Design review of the part built by this model. Coordinates are the model's own, in mm. Coordinates: 2 decimals unless noted, no trailing zeros. Loops run counter-clockwise (first coordinate to the right, second up) from the corner with the lowest first, then second, coordinate; pieces in that order, holes last. Notation, with made-up numbers: (79.5, 39.5) -> (96.5, 39.5) arc R12 ccw to (96.5, 52.5) -> close; hole circle Ø3 at (-18, 17.5). An arc over 180 degrees is marked (long way). One line per item, written item: value. Start each with the question number.
1. Insertion check: pin 1 (2 mm diameter, centred on y = 1.5, z = -86.5, fed in from -X); pin 2 (3 mm diameter, centred on x = 107, y = -1, fed in from -Z); pin 3 (3 mm diameter, centred on y = 1, z = 0, fed in from +X); pin 4 (1.8 mm diameter, centred on x = 64.87, z = 64.87, fed in from -Y). Each pin has a flat end and moves straight along its axis. Give the tip position at first contact, or say it passes through.
2. Add section C-C on y = 1.25. Give the number of separate pieces and of enclosed holes in the cut face, plus the area to 3 significant figures.
3. For probe 1 along Z at (x, y) = (-51.5, 0.75); probe 2 along Z at (x, y) = (33, -3); probe 3 along X at (y, z) = (0, 36.5), list the stretches that pass through material, from the lowest coordinate up.
4. Add section A-A on z = 55. Write out the cut boundary in (x, y) (3 decimals).
5. Add section B-B on x = -29. Write out the cut boundary in (y, z) (3 decimals), plus the area to 3 significant figures.
```python
from build123d import *

# Parameters (mm, degrees)
BOSS_EXTRUDE1_DEPTH          = 3.175
SKETCH2_W                    = 2.75
SKETCH2_H                    = 2.5
SKETCH2_H_2                  = 4
SKETCH2_W_2                  = 1.125
SKETCH2_H_3                  = 7.5
CUT_EXTRUDE1_DEPTH           = 230.978807609
CIRPATTERN1_COUNT            = 4
F_3_0_3_DIAMETER_HOLE1_D     = 3
F_8_0_8_DIAMETER_HOLE1_D     = 8
F_8_0_8_DIAMETER_HOLE1_DEPTH = 6.35


with BuildPart() as part:
    # Sketch1 → Boss-Extrude1 (new, symmetric)
    with BuildSketch(Plane(origin=(0, 0, 0), x_dir=(1, 0, 0), z_dir=(0, 1, 0))):
        with BuildLine():
            Line((88.388347648, 98.994949366), (64.667874078, 75.274475795))
            ThreePointArc((64.667874078, 75.274475795), (-70.171862751, 70.171862751), (-75.274475795, -64.667874078))
            Line((-75.274475795, -64.667874078), (-98.994949366, -88.388347648))
            Line((-98.994949366, -88.388347648), (-54.800775542, -132.582521472))
            ThreePointArc((-54.800775542, -132.582521472), (17.67766953, -162.604076401), (90.156114601, -132.582521472))
            Line((90.156114601, -132.582521472), (132.582521472, -90.156114601))
            ThreePointArc((132.582521472, -90.156114601), (162.604076401, -17.67766953), (132.582521472, 54.800775542))
            Line((132.582521472, 54.800775542), (88.388347648, 98.994949366))
        make_face()
        with BuildLine():
            Line((-7.5, -7.5), (-7.5, -83.903460262))
            ThreePointArc((-7.5, -83.903460262), (-59.565261034, -59.565261034), (-83.903460262, -7.5))
            Line((-83.903460262, -7.5), (-7.5, -7.5))
        make_face(mode=Mode.SUBTRACT)
        with BuildLine():
            ThreePointArc((83.903460262, -7.5), (59.565261034, -59.565261034), (7.5, -83.903460262))
            Line((7.5, -83.903460262), (7.5, -7.5))
            Line((7.5, -7.5), (83.903460262, -7.5))
        make_face(mode=Mode.SUBTRACT)
        with BuildLine():
            ThreePointArc((-64.667874078, -75.274475795), (0, -99.238), (64.667874078, -75.274475795))
            Line((64.667874078, -75.274475795), (95.45941546, -106.066017178))
            Line((95.45941546, -106.066017178), (79.549512883, -121.975919755))
            ThreePointArc((79.549512883, -121.975919755), (17.67766953, -147.604076401), (-44.194173824, -121.975919755))
            Line((-44.194173824, -121.975919755), (-77.781745931, -88.388347648))
            Line((-77.781745931, -88.388347648), (-64.667874078, -75.274475795))
        make_face(mode=Mode.SUBTRACT)
        with BuildLine():
            ThreePointArc((75.274475795, -64.667874078), (99.238, 0), (75.274475795, 64.667874078))
            Line((75.274475795, 64.667874078), (88.388347648, 77.781745931))
            Line((88.388347648, 77.781745931), (121.975919755, 44.194173824))
            ThreePointArc((121.975919755, 44.194173824), (147.604076401, -17.67766953), (121.975919755, -79.549512883))
            Line((121.975919755, -79.549512883), (106.066017178, -95.45941546))
            Line((106.066017178, -95.45941546), (75.274475795, -64.667874078))
        make_face(mode=Mode.SUBTRACT)
        with BuildLine():
            Line((-7.5, 7.5), (-83.903460262, 7.5))
            ThreePointArc((-83.903460262, 7.5), (-59.565261034, 59.565261034), (-7.5, 83.903460262))
            Line((-7.5, 83.903460262), (-7.5, 7.5))
        make_face(mode=Mode.SUBTRACT)
        with BuildLine():
            ThreePointArc((7.5, 83.903460262), (59.565261034, 59.565261034), (83.903460262, 7.5))
            Line((83.903460262, 7.5), (7.5, 7.5))
            Line((7.5, 7.5), (7.5, 83.903460262))
        make_face(mode=Mode.SUBTRACT)
    extrude(amount=BOSS_EXTRUDE1_DEPTH, both=True)

    # Sketch2 → Cut-Extrude1 (cut, symmetric)
    with BuildSketch(Plane(origin=(0, 0, 0), x_dir=(1, 0, 0), z_dir=(0, 1, 0))):
        with Locations((0, 86.488)):
            Rectangle(SKETCH2_W, SKETCH2_H)
        with Locations((0, 89.738)):
            Rectangle(SKETCH2_W, SKETCH2_H_2)
        with Locations((1.9375, 89.738)):
            Rectangle(SKETCH2_W_2, SKETCH2_H_2)
        with Locations((0, 95.488)):
            Rectangle(SKETCH2_W, SKETCH2_H_3)
        with Locations((-1.9375, 89.738)):
            Rectangle(SKETCH2_W_2, SKETCH2_H_2)
    cut_extrude1 = extrude(amount=CUT_EXTRUDE1_DEPTH, both=True, mode=Mode.SUBTRACT)

    # CirPattern1: Cut-Extrude1 ×4 about axis
    cirpattern1_axis = Axis((0, 0, 0), (0, 1, 0))
    for i in range(1, CIRPATTERN1_COUNT):
        add(cut_extrude1.rotate(cirpattern1_axis, i * 360 / CIRPATTERN1_COUNT), mode=Mode.SUBTRACT)

    # Ø3.0 (3) Diameter Hole1 (through all)
    with Locations(Plane(origin=(0, 3.175, 0), x_dir=(1, 0, 0), z_dir=(0, 1, 0))):
        with Locations((-64.868561892, -64.868561892), (0, 0), (-64.868561892, 64.868561892), (64.868561892, 64.868561892), (64.868561892, -64.868561892)):
            Hole(F_3_0_3_DIAMETER_HOLE1_D / 2)

    # Ø8.0 (8) Diameter Hole1
    with Locations(Plane(origin=(0, 3.175, 0), x_dir=(1, 0, 0), z_dir=(0, 1, 0))):
        with Locations((0, 0)):
            Hole(F_8_0_8_DIAMETER_HOLE1_D / 2, depth=F_8_0_8_DIAMETER_HOLE1_DEPTH)


solid = part.part
```
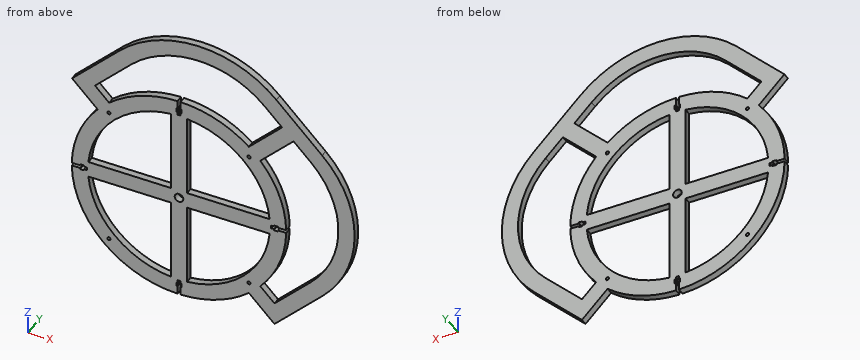
Worked answers:
1. pin 1: stops at x = -50.38
1. pin 2: stops at z = -81.88
1. pin 3: stops at x = 161.32
1. pin 4: passes through
2. separate pieces: 1
2. enclosed holes: 11
2. area: 21,700 mm²
3. probe 1: z = -84.83 to -66.66, -7.5 to 7.5, 66.66 to 84.83, 114.67 to 135.74
3. probe 2: z = -93.59 to -77.51, -7.5 to 7.5, 77.51 to 93.59, 146.25 to 161.45
3. probe 3: x = -92.28 to -75.92, -7.5 to 7.5, 75.92 to 92.28, 145.56 to 160.86
4. outline: (-82.603, -3.175) -> (-63.805, -3.175) -> (-63.805, 3.175) -> (-82.603, 3.175) -> close; (-7.5, -3.175) -> (7.5, -3.175) -> (7.5, 3.175) -> (-7.5, 3.175) -> close; (63.805, -3.175) -> (82.603, -3.175) -> (82.603, 3.175) -> (63.805, 3.175) -> close; (139.245, -3.175) -> (155.568, -3.175) -> (155.568, 3.175) -> (139.245, 3.175) -> close
5. outline: (-3.175, -94.906) -> (3.175, -94.906) -> (3.175, -79.089) -> (-3.175, -79.089) -> close; (-3.175, -7.5) -> (3.175, -7.5) -> (3.175, 7.5) -> (-3.175, 7.5) -> close; (-3.175, 79.089) -> (3.175, 79.089) -> (3.175, 94.906) -> (-3.175, 94.906) -> close; (-3.175, 134.114) -> (3.175, 134.114) -> (3.175, 151.359) -> (-3.175, 151.359) -> close
5. area: 406 mm²
